from build123d import *

# Parameters (mm, degrees)
SKETCH1_W                 = 19.84502
SKETCH1_H                 = 22.225
BODY_DEPTH                = 19.05
YAW_AXLE_OPENING_DEPTH    = 36.364925333
F_6_32_TAPPED_HOLE1_D     = 2.7051
F_6_32_TAPPED_HOLE1_DEPTH = 4.7625
F_6_32_TAPPED_HOLE1_TIP   = 0.81269403
F_6_32_TAPPED_HOLE2_D     = 2.7051
F_6_32_TAPPED_HOLE2_DEPTH = 4.7625
F_6_32_TAPPED_HOLE2_TIP   = 0.81269403
F_6_32_TAPPED_HOLE3_D     = 2.7051
F_6_32_TAPPED_HOLE3_DEPTH = 3.81
F_6_32_TAPPED_HOLE3_TIP   = 0.81269403
FILLET1_R                 = 1.27


with BuildPart() as part:
    # Sketch1 → Body (new body)
    with BuildSketch(Plane.XY):
        with Locations((9.92251, 11.1125)):
            Rectangle(SKETCH1_W, SKETCH1_H)
    extrude(amount=BODY_DEPTH)

    # Sketch2 → Yaw Axle Opening (cut, through all)
    with BuildSketch(Plane(origin=(0, 22.225, 0), x_dir=(1, 0, 0), z_dir=(0, 1, 0))):
        with BuildLine():
            ThreePointArc((13.89126, -9.525), (12.728840038, -6.718669962), (9.92251, -5.55625))
            Line((9.92251, -5.55625), (9.92251, -9.525))
            Line((9.92251, -9.525), (13.89126, -9.525))
        make_face()
        with BuildLine():
            Line((9.92251, -9.525), (9.92251, -5.55625))
            ThreePointArc((9.92251, -5.55625), (7.116179962, -6.718669962), (5.95376, -9.525))
            Line((5.95376, -9.525), (9.92251, -9.525))
        make_face()
        with BuildLine():
            Line((13.89126, -9.525), (9.92251, -9.525))
            Line((9.92251, -9.525), (9.92251, -13.49375))
            ThreePointArc((9.92251, -13.49375), (12.728840038, -12.331330038), (13.89126, -9.525))
        make_face()
        with BuildLine():
            Line((9.92251, -13.49375), (9.92251, -9.525))
            Line((9.92251, -9.525), (5.95376, -9.525))
            ThreePointArc((5.95376, -9.525), (7.116179962, -12.331330038), (9.92251, -13.49375))
        make_face()
    extrude(amount=-YAW_AXLE_OPENING_DEPTH, mode=Mode.SUBTRACT)

    # #6-32 Tapped Hole1
    with Locations(Plane(origin=(0, 17.4625, 9.525), x_dir=(0, 0, -1), z_dir=(-1, 0, 0))):
        with Locations((0, 0), (0, 12.7)):
            Hole(F_6_32_TAPPED_HOLE1_D / 2, depth=F_6_32_TAPPED_HOLE1_DEPTH)
            with Locations((0, 0, -(F_6_32_TAPPED_HOLE1_DEPTH + F_6_32_TAPPED_HOLE1_TIP / 2))):  # 118° drill point
                Cone(0, F_6_32_TAPPED_HOLE1_D / 2, F_6_32_TAPPED_HOLE1_TIP, mode=Mode.SUBTRACT)

    # #6-32 Tapped Hole2
    with Locations(Plane(origin=(19.84502, 17.4625, 9.525), x_dir=(0, 1, 0), z_dir=(1, 0, 0))):
        with Locations((0, 0), (-12.7, 0)):
            Hole(F_6_32_TAPPED_HOLE2_D / 2, depth=F_6_32_TAPPED_HOLE2_DEPTH)
            with Locations((0, 0, -(F_6_32_TAPPED_HOLE2_DEPTH + F_6_32_TAPPED_HOLE2_TIP / 2))):  # 118° drill point
                Cone(0, F_6_32_TAPPED_HOLE2_D / 2, F_6_32_TAPPED_HOLE2_TIP, mode=Mode.SUBTRACT)

    # #6-32 Tapped Hole3
    with Locations(Plane(origin=(0, 0, 0), x_dir=(-1, 0, 0), z_dir=(0, 0, -1))):
        with Locations((-9.92251, 17.225)):
            Hole(F_6_32_TAPPED_HOLE3_D / 2, depth=F_6_32_TAPPED_HOLE3_DEPTH)
            with Locations((0, 0, -(F_6_32_TAPPED_HOLE3_DEPTH + F_6_32_TAPPED_HOLE3_TIP / 2))):  # 118° drill point
                Cone(0, F_6_32_TAPPED_HOLE3_D / 2, F_6_32_TAPPED_HOLE3_TIP, mode=Mode.SUBTRACT)

    # Fillet1
    fillet1_edges = [part.edges().sort_by_distance(p)[0] for p in [
        (9.92251, 22.225, 19.05),
        (9.92251, 22.225, 0),
        (9.92251, 0, 0),
        (9.92251, 0, 19.05),
        (0, 22.225, 9.525),
        (19.84502, 22.225, 9.525),
        (19.84502, 0, 9.525),
        (0, 0, 9.525),
    ]]
    fillet(fillet1_edges, radius=FILLET1_R)


solid = part.part
Here's how the part is built. I have some questions about the finished solid (model axes, mm). A direction names the side the tool comes from. Give positions to 0.01 mm unless a question says otherwise; leave off trailing zeros. Loops run counter-clockwise (first coordinate to the right, second up) from the corner with the lowest first, then second, coordinate; pieces in that order, holes last. Notation, with made-up numbers: (-7.5, 24.5) -> (38.5, 24.5) arc R18 ccw to (38.5, 29.5) -> close; hole circle Ø4 at (43.25, 74.5). An arc over 180 degrees is marked (long way). Answer as a JSON object with one key per item and string values. Group by question number.
Item 1: Imagine slicing it at A-A on x = 15.75. Give the number of separate pieces and of enclosed holes in the cut face, then the cut area to 3 significant figures.
Item 2: Imagine slicing it at D-D on z = 6. Write out the boundary of the cut face in (x, y) (3 decimals), then the cut area to 3 significant figures.
Item 3: On a 3-axis mill with a long thin cutter (end or side, diameter ignored), from which of +Z, -Z, +X, -X, +Y, -Y can I reach the whole of each face in a straight line? I mean faces 1 (the cylindrical face through (2.41, 18.66, 10.15)), 2 (the cylindrical face through (10.5, 16, 1.9)), 3 (the cylindrical face through (10.061, 0.362, 18.668)). Say none if no direction works.
Item 4: Will these pins go through, and if not, where does the flat tip stop? pin 1 (2 mm diameter, centred on y = 17.46, z = 9.52, fed in from -X); pin 2 (2.5 mm diameter, centred on y = 17.46, z = 9.52, fed in from +X).
Item 5: Thinking about a two-plate mould opening in Y: for faces 4 (the cylindrical face through (19.463, 21.863, 9.658)), 5 (the flat face through (10, 11, 0)), 6 (the cylindrical face through (2.41, 3.62, 10.25)), 7 (the conical face through (5.434, 4.752, 9.76)), which applies, pulls with the +Y half, pulls with the -Y half, needs draft (parallel to the pull), parting line crosses it, or undercut?
Item 6: Imagine slicing it at B-B on z = 2. Write out the boundary of the cut face in (x, y) (3 decimals), then the cut area to 3 significant figures.
Item 7: I need wall thicknesses on L1, parallel to Y at x = 10, z = 1.5 (3 decimals); L2, parallel to X at y = 19, z = 9.5; L3, parallel to Z at x = 13.25, y = 21. Which ranges of each line are inside material? Lowest first, please.
Answer list:
{
 "1": {"separate pieces": "1", "enclosed holes": "2", "area": "411 mm2"},
 "2": {"outline": "(0, 1.27) arc R1.27 ccw to (1.27, 0) -> (8.099, 0) -> (8.099, 22.225) -> (1.27, 22.225) arc R1.27 ccw to (0, 20.955) -> close; (11.746, 0) -> (18.575, 0) arc R1.27 ccw to (19.845, 1.27) -> (19.845, 20.955) arc R1.27 ccw to (18.575, 22.225) -> (11.746, 22.225) -> close", "area": "359 mm2"},
 "3": {"face 1": "-X", "face 2": "-Z", "face 3": "+Z, +X, -X, -Y"},
 "4": {"pin 1": "stops at x = 4.97", "pin 2": "stops at x = 15.02"},
 "5": {"face 4": "pulls with the +Y half", "face 5": "needs draft", "face 6": "undercut", "face 7": "undercut"},
 "6": {"outline": "(0, 1.27) arc R1.27 ccw to (1.27, 0) -> (18.575, 0) arc R1.27 ccw to (19.845, 1.27) -> (19.845, 20.955) arc R1.27 ccw to (18.575, 22.225) -> (1.27, 22.225) arc R1.27 ccw to (0, 20.955) -> close; hole circle Ø2.705 at (9.923, 17.225)", "area": "434 mm2"},
 "7": {"L1": "y = 0 to 15.875, 18.575 to 22.225", "L2": "x = 0 to 5.95, 13.89 to 19.85", "L3": "z = 0 to 7.36, 11.69 to 19.05"}
}
